```python
from build123d import *

# Parameters (mm, degrees)
BOSS_EXTRUDE1_DEPTH                            = 6.35
CUT_EXTRUDE1_DEPTH                             = 7.35
CUT_EXTRUDE2_DEPTH                             = 7.35
FILLET1_R                                      = 2.54
CBORE_FOR_8_SOCKET_HEAD_CAP_SCREW1_D           = 4.9149
CBORE_FOR_8_SOCKET_HEAD_CAP_SCREW1_CBORE_D     = 7.9375
CBORE_FOR_8_SOCKET_HEAD_CAP_SCREW1_CBORE_DEPTH = 4.4196


with BuildPart() as part:
    # Sketch1 → Boss-Extrude1 (new body)
    with BuildSketch(Plane.XY):
        with BuildLine():
            Line((-19.668054922, 150.751853542), (-76.119138056, 0.215631852))
            ThreePointArc((-76.119138056, 0.215631852), (-76.179621009, -0.003695416), (-76.2, -0.230294919))
            Line((-76.2, -0.230294919), (-76.2, -3.81))
            ThreePointArc((-76.2, -3.81), (-75.828025612, -4.708025612), (-74.93, -5.08))
            Line((-74.93, -5.08), (-64.77, -5.08))
            ThreePointArc((-64.77, -5.08), (-63.871974388, -4.708025612), (-63.5, -3.81))
            Line((-63.5, -3.81), (-63.5, -1.27))
            ThreePointArc((-63.5, -1.27), (-63.128025612, -0.371974388), (-62.23, 0))
            Line((-62.23, 0), (62.23, 0))
            ThreePointArc((62.23, 0), (63.128025612, -0.371974388), (63.5, -1.27))
            Line((63.5, -1.27), (63.5, -3.81))
            ThreePointArc((63.5, -3.81), (63.871974388, -4.708025612), (64.77, -5.08))
            Line((64.77, -5.08), (74.93, -5.08))
            ThreePointArc((74.93, -5.08), (75.828025612, -4.708025612), (76.2, -3.81))
            Line((76.2, -3.81), (76.2, -0.230294919))
            ThreePointArc((76.2, -0.230294919), (76.179621009, -0.003695416), (76.119138056, 0.215631852))
            Line((76.119138056, 0.215631852), (19.668054922, 150.751853542))
            ThreePointArc((19.668054922, 150.751853542), (18.736549699, 151.947691069), (17.289778811, 152.4))
            Line((17.289778811, 152.4), (-17.289778811, 152.4))
            ThreePointArc((-17.289778811, 152.4), (-18.736549699, 151.947691069), (-19.668054922, 150.751853542))
        make_face()
    extrude(amount=BOSS_EXTRUDE1_DEPTH)

    # Sketch2 → Cut-Extrude1 (cut, through all)
    with BuildSketch(Plane(origin=(0, 0, 0), x_dir=(-1, 0, 0), z_dir=(0, 0, -1))):
        with BuildLine():
            Line((-8.859145886, 15.24), (-8.859145886, 122.164815439))
            ThreePointArc((-8.859145886, 122.164815439), (-10.94594688, 124.664057457), (-13.777421997, 123.056668981))
            Line((-13.777421997, 123.056668981), (-53.874227787, 16.131853542))
            ThreePointArc((-53.874227787, 16.131853542), (-53.583642745, 13.793229112), (-51.495951676, 12.7))
            Line((-51.495951676, 12.7), (-11.399145886, 12.7))
            ThreePointArc((-11.399145886, 12.7), (-9.603094662, 13.443948776), (-8.859145886, 15.24))
        make_face()
        with BuildLine():
            Line((53.874227787, 16.131853542), (13.777421997, 123.056668981))
            ThreePointArc((13.777421997, 123.056668981), (10.94594688, 124.664057457), (8.859145886, 122.164815439))
            Line((8.859145886, 122.164815439), (8.859145886, 15.24))
            ThreePointArc((8.859145886, 15.24), (9.603094662, 13.443948776), (11.399145886, 12.7))
            Line((11.399145886, 12.7), (51.495951676, 12.7))
            ThreePointArc((51.495951676, 12.7), (53.583642745, 13.793229112), (53.874227787, 16.131853542))
        make_face()
    extrude(amount=-CUT_EXTRUDE1_DEPTH, mode=Mode.SUBTRACT)

    # Sketch3 → Cut-Extrude2 (cut, through all)
    with BuildSketch(Plane(origin=(0, 0, 0), x_dir=(-1, 0, 0), z_dir=(0, 0, -1))):
        with BuildLine():
            Line((-6.35, 142.24), (-6.35, 152.4))
            Line((-6.35, 152.4), (6.35, 152.4))
            Line((6.35, 152.4), (6.35, 142.24))
            ThreePointArc((6.35, 142.24), (0, 135.89), (-6.35, 142.24))
        make_face()
    extrude(amount=-CUT_EXTRUDE2_DEPTH, mode=Mode.SUBTRACT)

    # Fillet1
    fillet1_edges = [part.edges().sort_by_distance(p)[0] for p in [
        (6.35, 152.4, 3.175),
        (-6.35, 152.4, 3.175),
    ]]
    fillet(fillet1_edges, radius=FILLET1_R)

    # CBORE for #8 Socket Head Cap Screw1 (through all)
    with Locations(Plane.XY.offset(6.35)):
        with Locations((-59.619847535, 22.511970393), (-64.079115243, 10.620589838), (59.619847535, 22.511970393), (64.079115243, 10.620589838)):
            CounterBoreHole(CBORE_FOR_8_SOCKET_HEAD_CAP_SCREW1_D / 2, CBORE_FOR_8_SOCKET_HEAD_CAP_SCREW1_CBORE_D / 2, CBORE_FOR_8_SOCKET_HEAD_CAP_SCREW1_CBORE_DEPTH)


solid = part.part
```
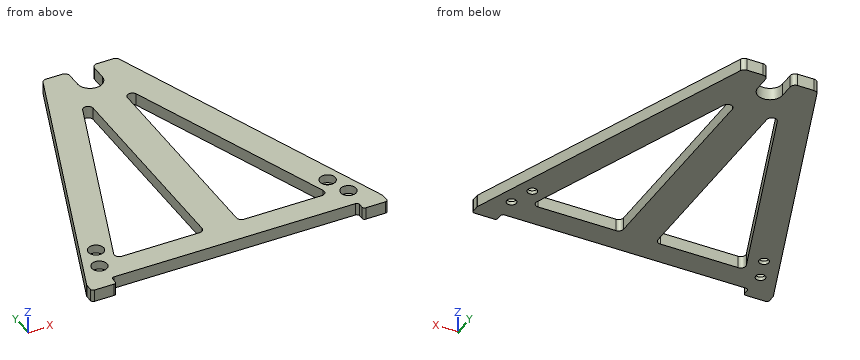
Build history of the part. All positions in model axes, mm. Round coordinates to 2 decimals unless told otherwise and drop trailing zeros. Write each loop counter-clockwise with the first axis right and the second up, starting at its lowest first coordinate (ties: lowest second). Pieces come first, ordered by that corner, then holes. Notation, with made-up numbers: (-12, 4) - (45, 4) arc R29 ccw to (45, 32) - close; hole circle Ø8 at (42.25, -38). An arc over 180 degrees is marked (long way). Write each question's results on one line, items separated by ' | '. Start each with the question number.
Item 1: Saw through at C-C (x = 0). Write the cut outline in (y, z), and give its area (3 significant figures).
Item 2: Wall check: L1, parallel to X at y = 28, z = 4; L2, parallel to X at y = 84.5, z = 1.25; L3, parallel to Y at x = 12.5, z = 1. Give the ranges that are in metal, low to high. Write a range as [from, to].
Item 3: Saw through at A-A (x = 33.5). Write the cut outline in (y, z), and give its area (3 significant figures).
Item 4: Drop flat-ended pins along their axis: P1, Ø5.5, axis at x = 59.62, y = 22.51, coming from the +Z side; P2, Ø2.5, axis at x = 65, y = 11, coming from the +Z side; P3, Ø1.9, axis at y = 148, z = 4, coming from the -X side; P4, Ø1, axis at x = -23, z = 1, coming from the -Y side. Give the stop position or say it passes through.
Item 5: Saw through at D-D (z = 3.25). State how many separate pieces and enclosed holes the cut face has, and give its area (3 significant figures).
Item 6: Saw through at B-B (y = 98.5). Write the cut outline in (x, z).
Results are:
1) outline: (0, 0) - (135.89, 0) - (135.89, 6.35) - (0, 6.35) - close | area: 863 mm²
2) L1: x = [-65.7, -49.42], [-8.86, 8.86], [49.42, 65.7] | L2: x = [-44.51, -28.24], [-8.86, 8.86], [28.24, 44.51] | L3: y = [0, 12.7], [124.45, 152.4]
3) outline: (0, 0) - (12.7, 0) - (12.7, 6.35) - (0, 6.35) - close; (70.46, 0) - (113.87, 0) - (113.87, 6.35) - (70.46, 6.35) - close | area: 356 mm²
4) P1: stops at z = 1.93 | P2: passes through | P3: stops at x = -21.06 | P4: stops at y = 0
5) separate pieces: 1 | enclosed holes: 6 | area: 8,600 mm²
6) outline: (-39.26, 0) - (-22.99, 0) - (-22.99, 6.35) - (-39.26, 6.35) - close; (-8.86, 0) - (8.86, 0) - (8.86, 6.35) - (-8.86, 6.35) - close; (22.99, 0) - (39.26, 0) - (39.26, 6.35) - (22.99, 6.35) - close
